Could you check a few things on this model? Use its own coordinates, in mm. Coordinates: 2 decimals unless noted, no trailing zeros. Order: outer loops, then holes, each group sorted by start corner. A loop starts at its lowest first (then second) coordinate and runs counter-clockwise, first axis right, second up. Notation, with made-up numbers: (7.25, 20) -> (29.25, 20) arc R14 cw to (29.25, 45) -> close; hole circle Ø9 at (38, -40). An arc over 180 degrees is marked (long way). Return JSON: item names as keys, results as strings. Group by question number.
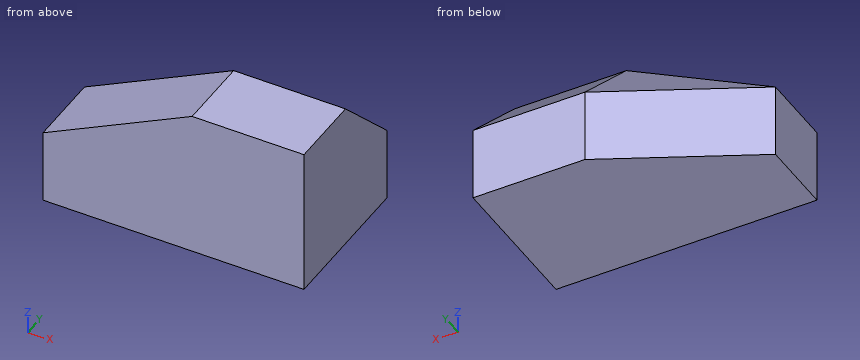
Autodesk Inventor part; units mm, degrees
ref_plane "YZ Plane" through (0, 0, 0) normal (1, 0, 0) x (0, 1, 0)
ref_plane "XZ Plane" through (0, 0, 0) normal (0, 1, 0) x (-1, 0, 0)
ref_plane "XY Plane" through (0, 0, 0) normal (0, 0, 1) x (1, 0, 0)
sketch "Sketch1" plane through (0, 0, 0) normal (0, 0, 1) x (1, 0, 0)
  line L0 (0, 0) -> (0, 20)
  line L1 (0, 20) -> (40, 40)
  line L2 (40, 40) -> (70, 40)
  line L3 (70, 40) -> (70, 0)
  line L4 (70, 0) -> (0, 0)
  dimension "d0" = 70
  dimension "d1" = 40
  dimension "d2" = 20
  dimension "d3" = 30
extrude "Extrusion1" add sketch "Sketch1" along normal blind 40
sketch "Sketch2" plane through (0, 0, 0) normal (0, -1, 0) x (1, 0, 0)
  line L0 (0, 40) -> (70, 40)
  line L1 (0, 0) -> (0, 40)
  line L2 (0, 0) -> (0, 40)
  line L3 (0, 20) -> (40, 40)
extrude "Extrusion2" cut sketch "Sketch2" against normal through all
sketch "Sketch3" plane through (70, 0, 0) normal (1, 0, 0) x (0, 0, -1)
  line L0 (0, 40) -> (-40, 40)
  line L1 (-40, 0) -> (-40, 40)
  line L2 (-20, 40) -> (-40, 20)
extrude "Extrusion3" cut sketch "Sketch3" against normal through all
sketch "Sketch4" plane through (40, 20, 40) normal (0, 0.7071, 0.7071) x (1, 0, 0)
  line L0 (-20, 14.1421) -> (0, 28.2843)
  line L1 (0, 0) -> (-20, 14.1421)
  line L2 (0, 28.2843) -> (0, 0)
  point P0 (-40, 14.1421)
sketch "Sketch5" plane through (0, 20, 20) normal (-0.4472, 0.8944, 0) x (0.8944, 0.4472, 0)
  line L0 (-8.9443, 0) -> (0, 0)
  line L1 (44.7214, 0) -> (0, 0)
  point P0 (-8.9443, 20)
sweep "Sweep1" cut profiles "Sketch4" path "Sketch5" path curves L1
properties part number "B7"
Q1. I want a section at A-A on y = 27.5. Please give me the cut outline in (x, z).
Q2. I want a section at B-B on x = 18. Please give me the cut outline in (y, z).
Q3. I need wall thicknesses on line 1 along X through (y, z) = (30, 11); line 2 along X through (y, z) = (15, 31); line 3 along Z through (x, y) = (28, 19). Which ranges of each line are inside material? Lowest first, please. Write a range as from..to.
Q4. I'm going to push flat-ended pins straight in: pin 1 Ø10 at (x, z) = (28, 11) entering from +Y; pin 2 Ø1 at (y, z) = (26.5, 6.5) entering from -X. Where does each tip first touch, or does it pass through?
Response values:
{
 "1": {"outline": "(15, 0) -> (70, 0) -> (70, 32.5) -> (40, 32.5) -> (15, 20) -> close"},
 "2": {"outline": "(0, 0) -> (29, 0) -> (29, 20) -> (20, 29) -> (0, 29) -> close"},
 "3": {"line 1": "x = 20..70", "line 2": "x = 22..70", "line 3": "z = 0..34"},
 "4": {"pin 1": "stops at y = 36.5", "pin 2": "stops at x = 12"}
}
